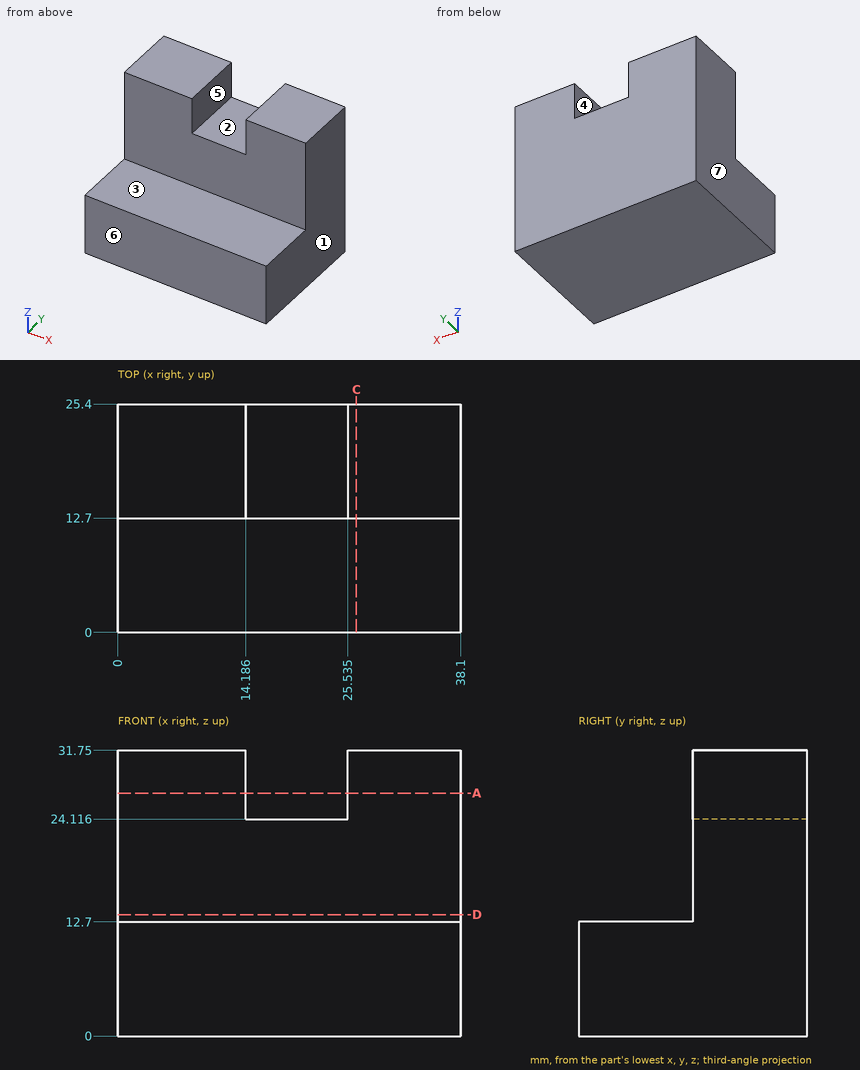
Design review of the part shown in the three views and the two pictorial views. Dimensions are in mm from the part's minimum x, y and z. A direction names the side the tool comes from. Coordinates: 2 decimals unless noted, no trailing zeros. Write each loop counter-clockwise with the first axis right and the second up, starting at its lowest first coordinate (ties: lowest second). Pieces come first, ordered by that corner, then holes.
1) Machinability: for the marked faces 1, 2 and 3, which of the approach directions +Z, -Z, +X, -X, +Y, -Y give a long, thin tool a straight path to every point of the face, cutting with its end or side? Answer none if there is none.
2) We need section C-C on x = 26.5. State the section outline as (y, z) points.
3) We need section D-D on z = 13.5. State the section outline as (x, y) points.
4) To check wall thickness, follow probe 1 along X at (y, z) = (12.75, 28.5) (1 decimal); probe 2 along Y at (x, z) = (7, 13); probe 3 along Z at (x, y) = (34.5, 9.25). State the ranges of each line that lie inside material, in increasing order.
5) Clearance check with flat-ended pins moving along their axes: pin 1 Ø9.5 at (x, z) = (18, 18.5) entering from -Y; pin 2 Ø2 at (y, z) = (20, 17) entering from -X; pin 3 Ø2 at (x, y) = (33, 8) entering from +Z; pin 4 Ø5.5 at (x, y) = (18, 22) entering from +Z. State where each tip first meets the part, or that it passes through.
6) We need section A-A on z = 27. State the section outline as (x, y) points (1 decimal).
7) The part is to be moulded in two halves that separate along X. For the marked faces 4, 5, 6 and 7, say which applies: pulls with the +X half, pulls with the -X half, needs draft (parallel to the pull), parting line crosses it, or undercut.
Answer list:
1. face 1: +Z, -Z, +X, +Y, -Y
1. face 2: +Z, +Y, -Y
1. face 3: +Z, +X, -X, -Y
2. outline: (0, 0) - (25.4, 0) - (25.4, 31.75) - (12.7, 31.75) - (12.7, 12.7) - (0, 12.7) - close
3. outline: (0, 12.7) - (38.1, 12.7) - (38.1, 25.4) - (0, 25.4) - close
4. probe 1: x = 0 to 14.2, 25.5 to 38.1
4. probe 2: y = 12.7 to 25.4
4. probe 3: z = 0 to 12.7
5. pin 1: stops at y = 12.7
5. pin 2: stops at x = 0
5. pin 3: stops at z = 12.7
5. pin 4: stops at z = 24.12
6. outline: (0, 12.7) - (14.2, 12.7) - (14.2, 25.4) - (0, 25.4) - close; (25.5, 12.7) - (38.1, 12.7) - (38.1, 25.4) - (25.5, 25.4) - close
7. face 4: undercut
7. face 5: undercut
7. face 6: needs draft
7. face 7: pulls with the -X half
